Geometry: see drawing. Coordinates: mm, zero at the bounding-box minimum. Give positions to 0.01 mm unless a question says otherwise; leave off trailing zeros. Write each loop counter-clockwise with the first axis right and the second up, starting at its lowest first coordinate (ties: lowest second). Pieces come first, ordered by that corner, then holes. Notation, with made-up numbers: (-30.5, 76) - (-15.5, 76) arc R15 cw to (-15.5, 105) - close; hole circle Ø10 at (5, -13.5). An arc over 180 degrees is marked (long way). Return JSON: item names as keys, results as strings.
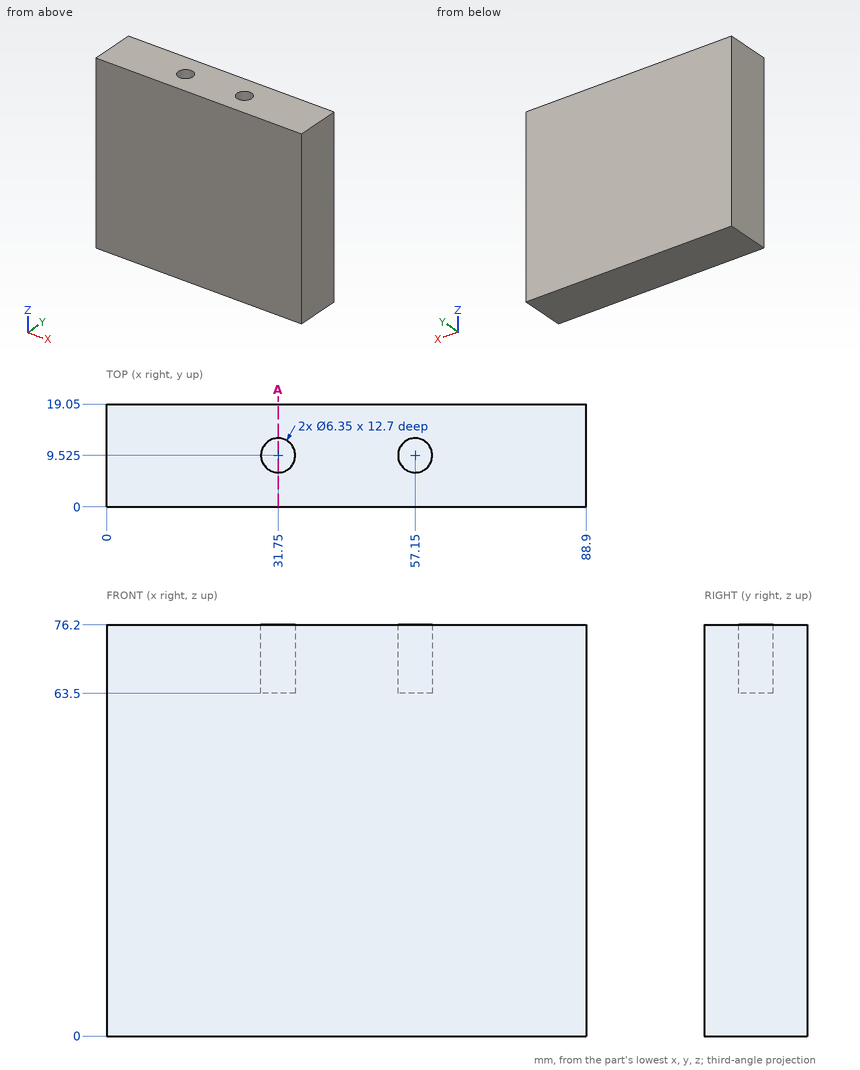
Q1. Section query A-A, the plane x = 31.75. Return the cut outline in (y, z).
Answer key:
{"outline": "(0, 0) - (19.05, 0) - (19.05, 76.2) - (12.7, 76.2) - (12.7, 63.5) - (6.35, 63.5) - (6.35, 76.2) - (0, 76.2) - close"}
Q2. Pin query (flat end, axial travel): P1, Ø1.9, axis at x = 30.5, y = 8, coming from the +Z side. Return the tip coordinate at first contact, or that it passes through.
Answer key:
{"P1": "stops at z = 63.5"}
Q3. Material intervals for probe 1 along Y at (x, z) = (57, 67); probe 2 along X at (y, z) = (11, 71); probe 3 along Y at (x, z) = (31, 69), sorted ascending. Write a range as [from, to].
Answer key:
{"probe 1": "y = [0, 6.35], [12.7, 19.05]", "probe 2": "x = [0, 28.94], [34.56, 54.34], [59.96, 88.9]", "probe 3": "y = [0, 6.44], [12.61, 19.05]"}
